Answer from the drawing. Dimensions are ordinates in mm from the lowest x, y and z of the part. Round coordinates to 2 decimals unless told otherwise and drop trailing zeros. Answer as a JSON object with one key per item and string values. Group by question number.
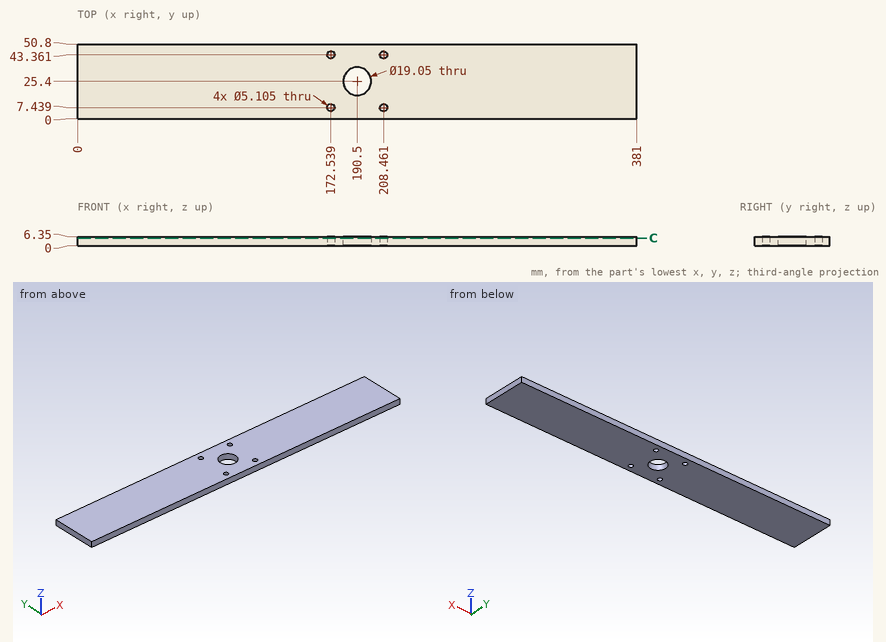
Item 1: Find section C-C (z = 5.25). Give the number of separate pieces and of enclosed holes in the cut face, and give its area (3 significant figures).
Item 2: Consider L1, parallel to Y at x = 190.5, z = 2.5 (1 decimal); L2, parallel to X at y = 42, z = 2.5; L3, parallel to X at y = 25.5, z = 1.25 (1 decimal). Determine where each line is inside the solid, lowest interval first.
Item 3: This flat-tipped pin is pushed along its axis until it touches: pin 1 (4.5 mm diameter, centred on x = 208.46, y = 43.36, fed in from +Z). Where does it stop, or does it pass through?
Responses:
{
 "1": {"separate pieces": "1", "enclosed holes": "5", "area": "19,000 mm^2"},
 "2": {"L1": "y = 0 to 15.9, 34.9 to 50.8", "L2": "x = 0 to 170.38, 174.7 to 206.3, 210.62 to 381", "L3": "x = 0 to 181, 200 to 381"},
 "3": {"pin 1": "passes through"}
}
